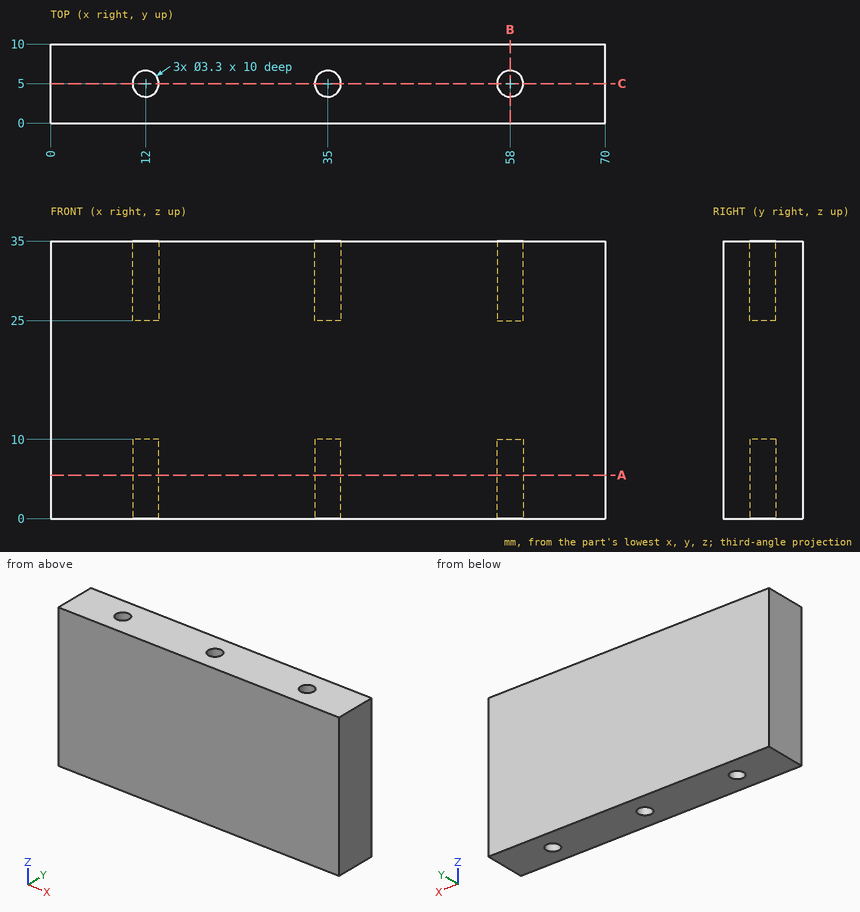
Print and shaded views of the part. All mm, measured from the part's lowest x, y and z. Coordinates: 2 decimals unless noted, no trailing zeros. Loops run counter-clockwise (first coordinate to the right, second up) from the corner with the lowest first, then second, coordinate; pieces in that order, holes last. Notation, with made-up numbers: M 64,21 L 70,21 A18 ccw 70,34 Z; hole C 51,46 d10. An arc over 180 degrees is marked long. Use a Markdown table: item, result. Add a question column.
Q1. Probe L1, parallel to Y at x = 12, z = 28.25; L2, parallel to Z at x = 34.5, y = 6.5. List the from-to ranges inside material, lowest first.
Q2. Pin check, flat tips, straight feed: P1, Ø2, axis at x = 58, y = 5, coming from the +Z side; P2, Ø1.6, axis at x = 35.5, y = 5.5, coming from the -Z side. Stop position of each tip, or through.
Q3. Cut at B-B (x = 58). Write the cut outline in (y, z).
Q4. Cut at C-C (y = 5). Write the cut outline in (x, z).
Q5. Cut at A-A (z = 5.5). Write the cut outline in (x, y), and give its area (3 significant figures).
Worked out:
| question | item | result |
|---|---|---|
| 1 | L1 | y = 0 to 3.35, 6.65 to 10 |
| 1 | L2 | z = 10 to 25 |
| 2 | P1 | stops at z = 25 |
| 2 | P2 | stops at z = 10 |
| 3 | outline | M 0,0 L 3.35,0 L 3.35,10 L 6.65,10 L 6.65,0 L 10,0 L 10,35 L 6.65,35 L 6.65,25 L 3.35,25 L 3.35,35 L 0,35 Z |
| 4 | outline | M 0,0 L 10.35,0 L 10.35,10 L 13.65,10 L 13.65,0 L 33.35,0 L 33.35,10 L 36.65,10 L 36.65,0 L 56.35,0 L 56.35,10 L 59.65,10 L 59.65,0 L 70,0 L 70,35 L 59.65,35 L 59.65,25 L 56.35,25 L 56.35,35 L 36.65,35 L 36.65,25 L 33.35,25 L 33.35,35 L 13.65,35 L 13.65,25 L 10.35,25 L 10.35,35 L 0,35 Z |
| 5 | outline | M 0,0 L 70,0 L 70,10 L 0,10 Z; hole C 12,5 d3.3; hole C 35,5 d3.3; hole C 58,5 d3.3 |
| 5 | area | 674 mm2 |
